Here's how the part is built. I have some questions about the finished solid (model axes, mm). A direction names the side the tool comes from. Round coordinates to 2 decimals unless told otherwise and drop trailing zeros. Write each loop counter-clockwise with the first axis right and the second up, starting at its lowest first coordinate (ties: lowest second). Pieces come first, ordered by that corner, then holes. Notation, with made-up numbers: (27, 13.25) - (55, 13.25) arc R27 cw to (55, 31.25) - close; hole circle Ø4 at (49, 70.25). An arc over 180 degrees is marked (long way). One line per question, with ' | ' between items. Start each with the question number.
(1) Imagine slicing it at A-A (x = 0). Write out the boundary of the cut face in (y, z), plus the area to 3 significant figures.
(2) Thinking about a two-plate mould opening in X: for faces 4 (the conical face through (-2.998, -48.125, -38.004)), 5 (the cylindrical face through (-1.665, -23.664, 34.736)), 6 (the flat face through (-1, 25, 1)), 7 (the cylindrical face through (-8.965, 12.325, -40.371)), which applies, pulls with the +X half, pulls with the -X half, needs draft (parallel to the pull), parting line crosses it, or undercut?
(3) Will these pins go through, and if not, where does the flat tip stop? pin 1 (6 mm diameter, centred on y = 14, z = -23.5, fed in from +X); pin 2 (8 mm diameter, centred on x = 26, y = -5.5, fed in from -Z); pin 3 (22 mm diameter, centred on x = 2.5, z = -28, fed in from -Y); pin 4 (10 mm diameter, centred on x = 36.5, z = -26.5, fed in from +Y).
(4) For faces 1 (the flat face through (-1, -50, 1)), 2 (the flat face through (-17, 0, -38)), 3 (the cylindrical face through (6.324, -23.664, -36.662)), which set-ups out of +Z, -Z, +X, -X, +Y, -Y let a thin tool reach every point of the face, with its end or its side?
(5) Imagine slicing it at B-B (z = 0). Write out the boundary of the cut face in (x, y).
(6) Imagine slicing it at C-C (y = 1.5). Write out the boundary of the cut face in (x, z).
(7) Imagine slicing it at D-D (y = -37.5). Write out the boundary of the cut face in (x, z).
(8) If I drill on L1, parallel to Z at x = 0, y = -13; L2, parallel to Z at x = -3, y = -8; L3, parallel to X at y = -26.5, z = 32.5, over which ranges is the centre line in solid material (lowest first)?
from build123d import *

# Parameters (mm, degrees)
F0_R     = 46.620662
F0_R_2   = 13.705086
F0_R_3   = 12.792455
F1_DEPTH = 50
F2_SIZE  = 2
F3_R     = 41.354393
F4_DEPTH = 25


with BuildPart() as f1:
    # F0 (on Front) → F1 (new body)
    with BuildSketch(Plane.XZ):
        Circle(F0_R)
        with Locations((0, -24.502814)):
            Circle(F0_R_2, mode=Mode.SUBTRACT)
        with Locations((0, 22.052526)):
            Circle(F0_R_3, mode=Mode.SUBTRACT)
    extrude(amount=F1_DEPTH)

    # F2
    f2_edges = [f1.edges().sort_by_distance(p)[0] for p in [
        (-46.620662, -50, 0),
        (-13.705086, -50, -24.502814),
        (-12.792455, -50, 22.052526),
    ]]
    chamfer(f2_edges, length=F2_SIZE)

    # F3 (on Front) → F4 (join)
    with BuildSketch(Plane.XZ):
        Circle(F3_R)
    extrude(amount=-F4_DEPTH)


solid = f1.part
Check sheet entries:
1) outline: (-50, -44.62) - (-48, -46.62) - (0, -46.62) - (0, -41.35) - (25, -41.35) - (25, 41.35) - (0, 41.35) - (0, 46.62) - (-48, 46.62) - (-50, 44.62) - (-50, 36.84) - (-48, 34.84) - (0, 34.84) - (0, 9.26) - (-48, 9.26) - (-50, 7.26) - (-50, -8.8) - (-48, -10.8) - (0, -10.8) - (0, -38.21) - (-48, -38.21) - (-50, -40.21) - close | area: 4,070 mm^2
2) face 4: undercut | face 5: undercut | face 6: needs draft | face 7: parting line crosses it
3) pin 1: x = 35.92 | pin 2: z = -41.1 | pin 3: y = -49.59 | pin 4: y = 25
4) face 1: +Z, -Z, +X, -X, -Y | face 2: +Y | face 3: -Y
5) outline: (-46.62, -48) - (-44.62, -50) - (44.62, -50) - (46.62, -48) - (46.62, 0) - (41.35, 0) - (41.35, 25) - (-41.35, 25) - (-41.35, 0) - (-46.62, 0) - close
6) outline: circle Ø82.71 at (0, 0)
7) outline: circle Ø93.24 at (0, 0); hole circle Ø27.41 at (0, -24.5); hole circle Ø25.58 at (0, 22.05)
8) L1: -46.62 to -38.21, -10.8 to 9.26, 34.84 to 46.62 | L2: -46.52 to -37.88, -11.13 to 9.62, 34.49 to 46.52 | L3: -33.43 to -7.38, 7.38 to 33.43
